Print and shaded views of the part. All mm, measured from the part's lowest x, y and z. Give positions to 0.01 mm unless a question says otherwise; leave off trailing zeros. Loops run counter-clockwise (first coordinate to the right, second up) from the corner with the lowest first, then second, coordinate; pieces in that order, holes last. Notation, with made-up numbers: (11.25, 79.5) - (43.25, 79.5) arc R9 cw to (43.25, 86.5) - close; hole circle Ø5 at (-11.75, 80). An arc over 180 degrees is marked (long way). Return JSON: item names as keys, results as strings.
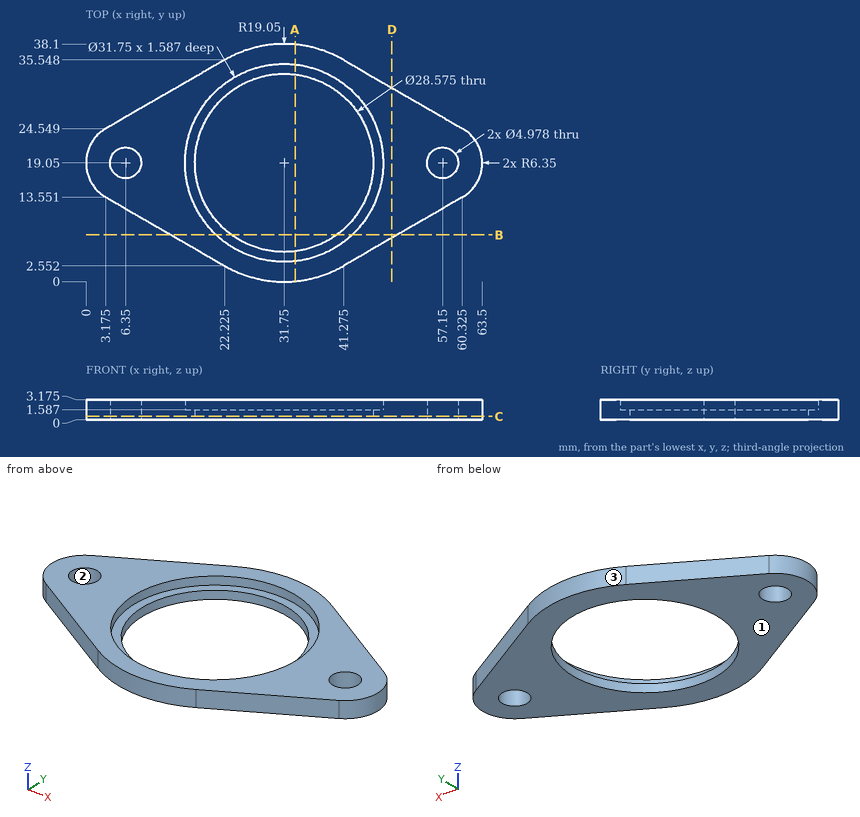
1. Pull direction X, two halves, no side cores. Call the marked faces 1, 2 and 3: +X half, -X half, draft (parallel to the pull), parting line (faces both ways), or undercut.
Values follow:
{"face 1": "draft", "face 2": "undercut", "face 3": "parting line"}
2. Cut at D-D, the plane x = 49. Write the cut outline in (y, z) (1 decimal).
Values follow:
{"outline": "(7, 0) - (31.1, 0) - (31.1, 3.2) - (7, 3.2) - close"}
3. Cut at B-B, the plane y = 7.5. Write the cut outline in (x, z) (1 decimal).
Values follow:
{"outline": "(13.7, 0) - (23.3, 0) - (23.3, 1.6) - (20.9, 1.6) - (20.9, 3.2) - (13.7, 3.2) - close; (40.2, 0) - (49.8, 0) - (49.8, 3.2) - (42.6, 3.2) - (42.6, 1.6) - (40.2, 1.6) - close"}
4. Cut at A-A, the plane x = 33.5. Write the cut outline in (y, z) (1 decimal).
Values follow:
{"outline": "(0.1, 0) - (4.9, 0) - (4.9, 1.6) - (3.3, 1.6) - (3.3, 3.2) - (0.1, 3.2) - close; (33.2, 0) - (38, 0) - (38, 3.2) - (34.8, 3.2) - (34.8, 1.6) - (33.2, 1.6) - close"}
5. Drop flat-ended pins along their axis: P1, Ø1.5, axis at y = 14.5, z = 1, coming from the -X side; P2, Ø5, axis at x = 55, y = 6.5, coming from the -Z side; P3, Ø2, axis at x = 19.5, y = 25.5, coming from the +Z side. Give the stop position or say it passes through.
Values follow:
{"P1": "stops at x = 1.26", "P2": "passes through", "P3": "stops at z = 1.59"}
6. Cut at C-C, the plane z = 0.5. Give the number of separate pieces and of enclosed holes in the cut face.
Values follow:
{"separate pieces": "1", "enclosed holes": "3"}
7. Drill centre lines: probe 1 along X at (y, z) = (18, 2.25) (1 decimal); probe 2 along X at (y, z) = (30, 2.7) (1 decimal); probe 3 along X at (y, z) = (5.5, 2.8) (1 decimal). Where is each one in solid material? Low to high.
Values follow:
{"probe 1": "x = 0.1 to 4.1, 8.6 to 15.9, 47.6 to 54.9, 59.4 to 63.4", "probe 2": "x = 12.6 to 20.3, 43.2 to 50.9", "probe 3": "x = 17.1 to 23.5, 40 to 46.4"}
